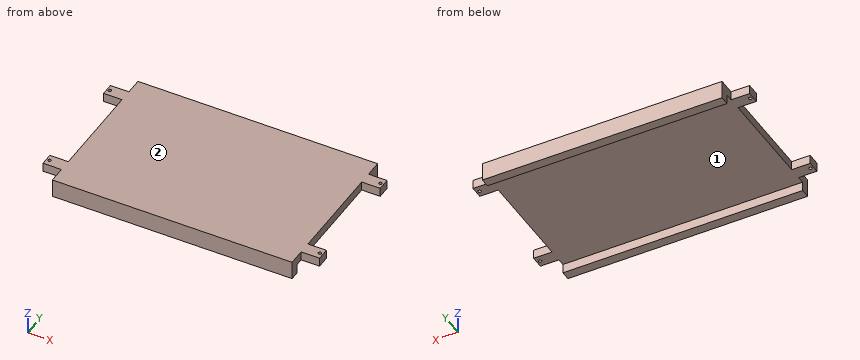
```python
from build123d import *

# Parameters (mm, degrees)
F1_DEPTH = 4.9
F2_R     = 0.85
F3_DEPTH = 4.901
F4_W     = 130
F4_H     = 4
F5_DEPTH = 4.9
F6_W     = 130
F6_H     = 5
F7_DEPTH = 10


with BuildPart() as f1:
    # F0 (on Top) → F1 (new body)
    with BuildSketch(Plane.XY):
        Polygon((-75, -33.5), (75, -33.5), (75, -26.7), (65, -26.7), (65, 26.7), (75, 26.7), (75, 33.5), (-75, 33.5), (-75, 26.7), (-65, 26.7), (-65, -26.7), (-75, -26.7), align=None)
    extrude(amount=F1_DEPTH)

    # F2 (on face) → F3 (cut, through all)
    with BuildSketch(Plane.XY.offset(4.9)):
        with Locations((-73.5, 30.1)):
            Circle(F2_R)
        with Locations((-73.3, -30.1)):
            Circle(F2_R)
        with Locations((73.3, 30.1)):
            Circle(F2_R)
        with Locations((73.3, -30.1)):
            Circle(F2_R)
    extrude(amount=-F3_DEPTH, mode=Mode.SUBTRACT)

    # F4 (on face) → F5 (join)
    with BuildSketch(Plane.XY.offset(4.9)):
        with Locations((0, 35.5)):
            Rectangle(F4_W, F4_H)
        with Locations((0, -35.5)):
            Rectangle(F4_W, F4_H)
    extrude(amount=-F5_DEPTH)

    # F6 (on face) → F7 (join)
    with BuildSketch(Plane.XY.offset(4.9)):
        with Locations((0, 40)):
            Rectangle(F6_W, F6_H)
        with Locations((0, -40)):
            Rectangle(F6_W, F6_H)
    extrude(amount=-F7_DEPTH)


solid = f1.part
```
Input: part model. Units: mm. Frame: model coordinates. Face numbers are marked on the shaded views. Coordinates: 2 decimals unless noted, no trailing zeros. Order: outer loops, then holes, each group sorted by start corner. A loop starts at its lowest first (then second) coordinate and runs counter-clockwise, first axis right, second up. Notation, with made-up numbers: (55.25, 57) - (78.25, 57) arc R26 ccw to (78.25, 75) - close; hole circle Ø2 at (-9.5, 16.25). An arc over 180 degrees is marked (long way). Return JSON: item names as keys, results as strings.
Q1. Ray query, probe 1 along Y at (x, z) = (73.3, 3.9); probe 2 along Y at (x, z) = (13, -2); probe 3 along Z at (x, y) = (-14.5, 10.5). Return the intervals inside material, ascending.
The answers:
{"probe 1": "y = -33.5 to -30.95, -29.25 to -26.7, 26.7 to 29.25, 30.95 to 33.5", "probe 2": "y = -42.5 to -37.5, 37.5 to 42.5", "probe 3": "z = 0 to 4.9"}
Q2. Cut plane A-A (z = 2.5). Return loops of the section in (x, y), then the cut area to 3 significant figures.
The answers:
{"outline": "(-75, -33.5) - (-65, -33.5) - (-65, -42.5) - (65, -42.5) - (65, -33.5) - (75, -33.5) - (75, -26.7) - (65, -26.7) - (65, 26.7) - (75, 26.7) - (75, 33.5) - (65, 33.5) - (65, 42.5) - (-65, 42.5) - (-65, 33.5) - (-75, 33.5) - (-75, 26.7) - (-65, 26.7) - (-65, -26.7) - (-75, -26.7) - close; hole circle Ø1.7 at (-73.5, 30.1); hole circle Ø1.7 at (-73.3, -30.1); hole circle Ø1.7 at (73.3, -30.1); hole circle Ø1.7 at (73.3, 30.1)", "area": "11,300 mm2"}
Q3. Cut plane B-B (x = -19.5). Return loops of the section in (y, z), then the cut area to 4 significant figures.
The answers:
{"outline": "(-42.5, -5.1) - (-37.5, -5.1) - (-37.5, 0) - (37.5, 0) - (37.5, -5.1) - (42.5, -5.1) - (42.5, 4.9) - (-42.5, 4.9) - close", "area": "467.5 mm2"}
Q4. Draft query along Y for the marked faces 1 and 2. Return one class per face: +Y half, -Y half, draft (parallel to the pull), parting line (faces both ways), or undercut.
The answers:
{"face 1": "undercut", "face 2": "draft"}
Q5. First-contact query: pin 1 (2.5 mm diameter, centred on y = 8.5, z = 2.5, fed in from -X); pin 2 (22.5 mm diameter, centred on x = -22, y = 16, fed in from -Z); pin 3 (4 mm diameter, centred on x = 70, z = 1.5, fed in from -Y). Flat tips, straight axial feed; report the tip coordinate or a pass-through.
The answers:
{"pin 1": "stops at x = -65", "pin 2": "stops at z = 0", "pin 3": "stops at y = -33.5"}
Q6. Cut plane C-C (y = -19.5). Return loops of the section in (x, z), then the cut area to 3 significant figures.
The answers:
{"outline": "(-65, 0) - (65, 0) - (65, 4.9) - (-65, 4.9) - close", "area": "637 mm2"}
